Input: part model. Units: mm. Frame: model coordinates. Coordinates: 2 decimals unless noted, no trailing zeros. Order: outer loops, then holes, each group sorted by start corner. A loop starts at its lowest first (then second) coordinate and runs counter-clockwise, first axis right, second up. Notation, with made-up numbers: M -28.75,41.5 L -14.75,41.5 A14 ccw -14.75,64.5 Z; hole C 49,-21.5 d3. An arc over 180 degrees is marked long. One line per item, written item: value.
```python
from build123d import *

# Parameters (mm, degrees)
F1_R     = 16.3135462342
F2_DEPTH = 46.736
F4_R     = 35.56


# Not quite as in the source:
# - an extrude whose draft closes it to a point is written as a loft to that point


with BuildPart() as f2:
    # F1 (on face) → F2 (new body)
    with BuildSketch(Plane.XY):
        Circle(F1_R)
    extrude(amount=F2_DEPTH)

    # F1 (on face) → F3 section 0
    with BuildSketch(Plane.XY, mode=Mode.PRIVATE) as f3_s0:
        Circle(F1_R)
    loft([f3_s0.sketch, Vertex(0, 0, -16.3135462342)], ruled=True)

    # F4
    f4_edges = [f2.edges().sort_by_distance(p)[0] for p in [
        (-16.313546, 0, 0),
    ]]
    fillet(f4_edges, radius=F4_R)


solid = f2.part
```
(1) First-contact query: pin 1 (2 mm diameter, centred on y = 4, z = 23, fed in from +X); pin 2 (10 mm diameter, centred on x = 6.5, z = -9, fed in from -Y); pin 3 (10 mm diameter, centred on x = 0.5, y = -9, fed in from -Z). Flat tips, straight axial feed; report the tip coordinate or a pass-through.
Data:
pin 1: stops at x = 16.04
pin 2: stops at y = -9.77
pin 3: stops at z = -12.3
(2) Cut plane A-A on z = 24. Output: boundary loops of the cut face in (x, y), plus the area to 3 significant figures.
Data:
outline: C 0,0 d32.63
area: 836 mm2
(3) Ray query, line 1 (Z direction, x = -2.5, y = 3); line 2 (X direction, y = -5, z = 26.5); line 3 (Z direction, x = -9.5, y = -9). Return the intervals inside material, ascending. Write a range as from..to.
Data:
line 1: z = -12.41..46.74
line 2: x = -15.53..15.53
line 3: z = -0.07..46.74
